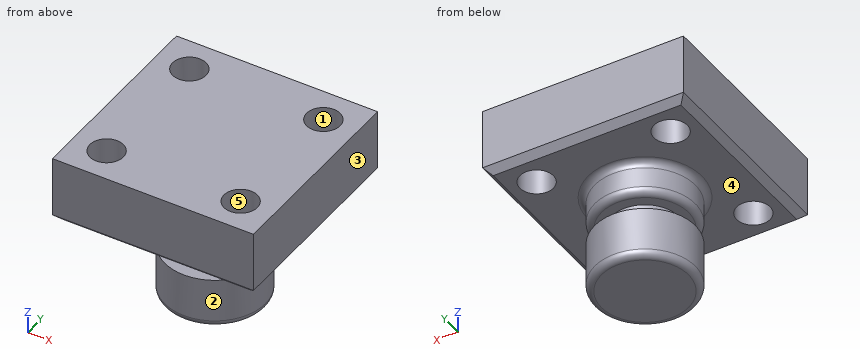
from build123d import *

# Parameters (mm, degrees)
F0_W     = 76.2
F0_H     = 76.2
F1_DEPTH = 25.4
F2_R     = 6.35
F3_DEPTH = 25.4
F4_R     = 6.35
F5_DEPTH = 25.4
F6_W     = 19.05
F6_H     = 38.1
F8_W     = 8.2727996377
F8_H     = 6.35
F10_SIZE = 2.54
F11_R    = 2.54


with BuildPart() as f1:
    # F0 (on Top) → F1 (new body)
    with BuildSketch(Plane.XY):
        Rectangle(F0_W, F0_H)
    extrude(amount=F1_DEPTH)

    # F2 (on face) → F3 (cut)
    with BuildSketch(Plane.XY.offset(25.4)):
        with Locations((25.4, 25.4)):
            Circle(F2_R)
        with Locations((25.4, -25.4)):
            Circle(F2_R)
        with Locations((-25.4, -25.4)):
            Circle(F2_R)
    extrude(amount=-F3_DEPTH, mode=Mode.SUBTRACT)

    # F4 (on face) → F5 (cut)
    with BuildSketch(Plane(origin=(0, 0, 0), x_dir=(1, 0, 0), z_dir=(0, 0, -1))):
        with Locations((-25.4, -25.4)):
            Circle(F4_R)
    extrude(amount=-F5_DEPTH, mode=Mode.SUBTRACT)

    # F6 (on Front) → F7 (revolve)
    with BuildSketch(Plane.XZ):
        with Locations((9.525, -19.05)):
            Rectangle(F6_W, F6_H)
    revolve(axis=Axis((0, 0, -19.05), (0, 0, 1)))

    # F8 (on Right) → F9 (revolve, cut)
    with BuildSketch(Plane.YZ):
        with Locations((-16.8363998188, -15.875)):
            Rectangle(F8_W, F8_H)
    revolve(axis=Axis((0, 0, -38.1), (0, 0, 1)), mode=Mode.SUBTRACT)

    # F10
    f10_edges = [f1.edges().sort_by_distance(p)[0] for p in [
        (-38.1, 0, 0),
        (0, 38.1, 0),
        (38.1, 0, 0),
        (0, -38.1, 0),
    ]]
    chamfer(f10_edges, length=F10_SIZE)

    # F11
    f11_edges = [f1.edges().sort_by_distance(p)[0] for p in [
        (-19.05, 0, -12.7),
        (-19.05, 0, 0),
        (-19.05, 0, -38.1),
    ]]
    fillet(f11_edges, radius=F11_R)


solid = f1.part
Verification items for the finished model (mm, model axes). Face numbers are marked on the shaded views. A direction names the side the tool comes from. Coordinates: 2 decimals unless noted, no trailing zeros. Order: outer loops, then holes, each group sorted by start corner. A loop starts at its lowest first (then second) coordinate and runs counter-clockwise, first axis right, second up.
1. Scan lines: line 1 (Y direction, x = -25.4, z = 10.75); line 2 (X direction, y = -25, z = 12); line 3 (Y direction, x = 20.5, z = 9). Record each from-to range of solid material in increasing order.
Results found:
line 1: y = -38.1 to -31.75, -19.05 to 19.05, 31.75 to 38.1
line 2: x = -38.1 to -31.74, -19.06 to 19.06, 31.74 to 38.1
line 3: y = -38.1 to -29.44, -21.36 to 21.36, 29.44 to 38.1
2. Release check for a two-part mould opening along Y. For the marked faces 1, 2 and 3 record: +Y half, -Y half, draft (parallel to the pull), parting line (faces both ways), or undercut.
Results found:
face 1: undercut
face 2: parting line
face 3: draft
3. Sectioned sample at D-D, the plane y = 0. Record the cut outline in (x, z).
Results found:
outline: (-38.1, 2.54) - (-35.56, 0) - (-21.59, 0) arc R2.54 cw to (-19.05, -2.54) - (-19.05, -10.16) arc R2.54 ccw to (-16.51, -12.7) - (-12.7, -12.7) - (-12.7, -19.05) - (-19.05, -19.05) - (-19.05, -35.56) arc R2.54 ccw to (-16.51, -38.1) - (16.51, -38.1) arc R2.54 ccw to (19.05, -35.56) - (19.05, -19.05) - (12.7, -19.05) - (12.7, -12.7) - (16.51, -12.7) arc R2.54 ccw to (19.05, -10.16) - (19.05, -2.54) arc R2.54 cw to (21.59, 0) - (35.56, 0) - (38.1, 2.54) - (38.1, 25.4) - (-38.1, 25.4) - close
4. Set-up check for the marked faces 4 and 5: record each of +Z, -Z, +X, -X, +Y, -Y from which the full face is reachable in a straight line by a thin tool's end or side.
Results found:
face 4: -Z
face 5: +Z, -Z
5. Sectioned sample at A-A, the plane y = -25.4. Record the cut outline in (x, z), and give its area (3 significant figures).
Results found:
outline: (-38.1, 2.54) - (-35.56, 0) - (-31.75, 0) - (-31.75, 25.4) - (-38.1, 25.4) - close; (-19.05, 0) - (19.05, 0) - (19.05, 25.4) - (-19.05, 25.4) - close; (31.75, 0) - (35.56, 0) - (38.1, 2.54) - (38.1, 25.4) - (31.75, 25.4) - close
area: 1,280 mm2
6. Go/stop test with flat-tipped pins: pin 1 Ø4 at (y, z) = (-15, -9) entering from +X; pin 2 Ø16.5 at (x, y) = (25.4, 25.4) entering from -Z; pin 3 Ø10 at (x, z) = (-8, -26.5) entering from +Y. Record where each tip stops, or that it passes through.
Results found:
pin 1: stops at x = 13.92
pin 2: stops at z = 0
pin 3: stops at y = 18.81
7. Sectioned sample at C-C, the plane z = 18.5. Record the cut outline in (x, y), and give its area (3 significant figures).
Results found:
outline: (-38.1, -38.1) - (38.1, -38.1) - (38.1, 38.1) - (-38.1, 38.1) - close; hole circle Ø12.7 at (-25.4, -25.4); hole circle Ø12.7 at (-25.4, 25.4); hole circle Ø12.7 at (25.4, -25.4); hole circle Ø12.7 at (25.4, 25.4)
area: 5,300 mm2
